Check sheet for the modelled part. Datum: model origin and axes. Units: mm. Face numbers are marked on the shaded views. Coordinates: 2 decimals unless noted, no trailing zeros. Loops run counter-clockwise (first coordinate to the right, second up) from the corner with the lowest first, then second, coordinate; pieces in that order, holes last. Notation, with made-up numbers: (-20.75, 40.25) -> (-0.75, 40.25) arc R5 ccw to (-0.75, 47.25) -> close; hole circle Ø7 at (-22.75, 12). An arc over 180 degrees is marked (long way). Use CSV: the item, a comma, the result in double quotes. Start each with the question number.
1. Release check for a two-part mould opening along Z. For the marked faces 1 and 2 record: pulls with the +Z half, pulls with the -Z half, needs draft (parallel to the pull), parting line crosses it, or undercut.
2. Thickness scan on L1, parallel to Y at x = 74.5, z = -3.5; L2, parallel to X at y = 9, z = -8.5; L3, parallel to Y at x = 258.5, z = -29. Record the ranges inside material, lowest first.
3. Sectioned sample at A-A, the plane z = 0. Record the cut outline in (x, y), and give its area (3 significant figures).
4. Sectioned sample at B-B, the plane z = 28. Record the cut outline in (x, y), and give its area (3 significant figures).
5. Sectioned sample at C-C, the plane z = 14.5. Record the cut outline in (x, y).
6. Gauge pin test, flat ends, axial feed: pin 1 (2 mm diameter, centred on x = 122.5, z = -4.5, fed in from -Y); pin 2 (8 mm diameter, centred on x = 155, y = -18.5, fed in from -Z); pin 3 (20 mm diameter, centred on x = 239.5, z = 15.5, fed in from -Y). Record the tip position at first contact, or that the pin passes through.
```python
from build123d import *

# Parameters (mm, degrees)
F1_R          = 6.35
F3_R          = 33.2925149607
F4_DEPTH      = 12.7
F4_DEPTH_BACK = 12.7
F5_R          = 11.3838907511
F6_DEPTH      = 25.4


with BuildPart() as f2:
    # F2: sweep along a path in F0
    with BuildLine(Plane.XY) as f2_path:
        Line((0, 68.0590948775), (0, -68.0590948775))
        Line((0, -68.0590948775), (254, 0))
        Line((254, 0), (0, 68.0590948775))
    # F1 (on Front) → F2 (sweep)
    with BuildSketch(Plane.XZ):
        Circle(F1_R)
    sweep(path=f2_path.line, transition=Transition.RIGHT)

    # F3 (on Front) → F4 (join, two sides)
    with BuildSketch(Plane.XZ) as f4_sk:
        with Locations((247.0585107803, 0)):
            Circle(F3_R)
    extrude(amount=F4_DEPTH)
    extrude(f4_sk.sketch, amount=-F4_DEPTH_BACK)

    # F5 (on face) → F6 (cut)
    with BuildSketch(Plane(origin=(0, 12.7, 0), x_dir=(-1, 0, 0), z_dir=(0, 1, 0))):
        with Locations((-247.0585107803, 0)):
            Circle(F5_R)
    extrude(amount=-F6_DEPTH, mode=Mode.SUBTRACT)


solid = f2.part
```
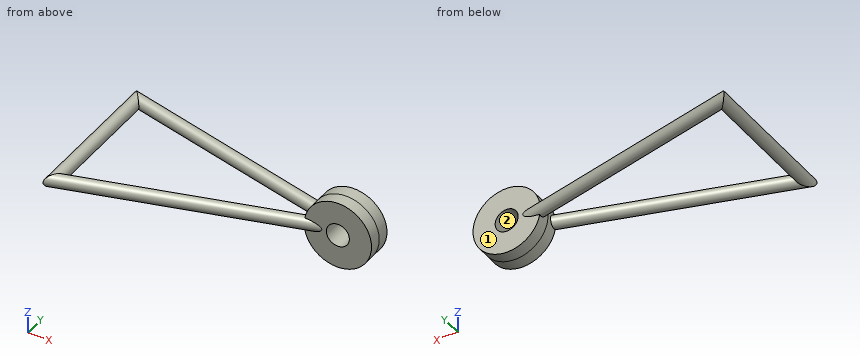
Completed:
1,face 1,"needs draft"
1,face 2,"undercut"
2,L1,"-53.58 to -42.61, 42.61 to 53.58"
2,L2,"214.87 to 239.49, 254.63 to 279.25"
2,L3,"-12.7 to 12.7"
3,outline,"(-6.35, -76.33) -> (231.14, -12.7) -> (235.67, -12.7) -> (235.67, 12.7) -> (231.14, 12.7) -> (-6.35, 76.33) -> close; (258.44, -12.7) -> (280.35, -12.7) -> (280.35, 12.7) -> (258.44, 12.7) -> close; hole (6.35, -59.78) -> (213.77, -4.21) -> (213.77, 4.21) -> (6.35, 59.78) -> close"
3,area,"8,540 mm²"
4,outline,"(229.05, -12.7) -> (265.07, -12.7) -> (265.07, 12.7) -> (229.05, 12.7) -> close"
4,area,"915 mm²"
5,outline,"(217.09, -12.7) -> (277.03, -12.7) -> (277.03, 12.7) -> (217.09, 12.7) -> close"
6,pin 1,"y = -40.77"
6,pin 2,"z = -5.12"
6,pin 3,"y = -12.7"
